For this review, take the finished solid that the model builds, in its own axes (mm). A direction names the side the tool comes from. Round coordinates to 2 decimals unless told otherwise and drop trailing zeros. Loops run counter-clockwise (first coordinate to the right, second up) from the corner with the lowest first, then second, coordinate; pieces in that order, holes last.
1) Take a section at B-B (z = -58). State the section outline as (x, y) points (3 decimals).
2) Take a section at C-C (x = 31). State the section outline as (y, z) points.
3) Insertion check: pin 1 (3 mm diameter, centred on x = -6, y = 27.5, fed in from +Z); pin 2 (8 mm diameter, centred on y = -0.5, z = -64, fed in from -X); pin 3 (3 mm diameter, centred on x = -1, z = -66, fed in from -Y). Each pin has a flat end and moves straight along its axis. Give the tip position at first contact, or say it passes through.
4) Tool access review of faces 1 (the cylindrical face through (-26, 0, 5)), 2 (the flat face through (5.25, 0, -65)), 3 (the flat face through (0, -5.25, -65)), 4 (the flat face through (-5.25, 0, -65)): name each direction out of +Z, -Z, +X, -X, +Y, -Y from which nothing blocks a thin tool from reaching the whole face with its end or side.
5) Take a section at D-D (z = 20.5). State the section outline as (x, y) points, then the cut area to 3 significant figures.
6) Mouldability with a two-part tool opening along Y and no side actions: class faces 5 (the flat face through (-24, -38, 55)), 6 (the flat face through (0, 0, -60.1)), 7 (the cylindrical face through (47.23, -1.34, 32.18)) as pulls with the +Y half, pulls with the -Y half, needs draft (parallel to the pull), parting line crosses it, or undercut.
```python
from build123d import *
from build123d.topology import SkipClean

# Parameters (mm, degrees)
SKETCH1_R           = 57
SKETCH1_R_2         = 5.175
BOSS_EXTRUDE1_DEPTH = 10
SKETCH3_R           = 2.25
BOSS_EXTRUDE2_DEPTH = 45
BOSS_EXTRUDE3_START = 60.1
SKETCH4_R           = 9.75
SKETCH4_R_2         = 5.175
BOSS_EXTRUDE3_DEPTH = 60.1
SKETCH5_W           = 10.5
SKETCH5_H           = 10.5
BOSS_EXTRUDE4_DEPTH = 10
CUT_EXTRUDE1_DEPTH  = 10
CIRPATTERN1_COUNT   = 3


with BuildPart() as part:
    # Sketch1 → Boss-Extrude1 (new body)
    with BuildSketch(Plane(origin=(0, 0, 0), x_dir=(0, 1, 0), z_dir=(0, 0, 1))):
        with Locations(Location((0, 0, 0), (0, 0, 270))):
            Circle(SKETCH1_R)
        with Locations(Location((0, 0, 0), (0, 0, 270))):
            Circle(SKETCH1_R_2, mode=Mode.SUBTRACT)
    extrude(amount=BOSS_EXTRUDE1_DEPTH)

    # Sketch3 → Boss-Extrude2 (add)
    with BuildSketch(Plane.XY.offset(10)):
        with Locations(Location((-21.418860984, 39.575654059, 0), (0, 0, 180))):
            Circle(SKETCH3_R)
    boss_extrude2 = extrude(amount=BOSS_EXTRUDE2_DEPTH)

    # Sketch4 → Boss-Extrude3 (add)
    with SkipClean():  # the faces are left unmerged after this step: merging them gives an invalid solid
        with BuildSketch(Plane(origin=(0, 0, 0), x_dir=(-1, 0, 0), z_dir=(0, 0, -1)).offset(BOSS_EXTRUDE3_START)):
            with Locations(Location((0, 0, 0), (0, 0, 180))):
                Circle(SKETCH4_R)
            Circle(SKETCH4_R_2, mode=Mode.SUBTRACT)
        extrude(amount=-BOSS_EXTRUDE3_DEPTH)

    # Sketch5 → Boss-Extrude4 (add)
    with SkipClean():  # the faces are left unmerged after this step: merging them gives an invalid solid
        with BuildSketch(Plane(origin=(0, 0, -60.1), x_dir=(-1, 0, 0), z_dir=(0, 0, -1))):
            Rectangle(SKETCH5_W, SKETCH5_H)
        extrude(amount=BOSS_EXTRUDE4_DEPTH)

    # Sketch6 → Cut-Extrude1 (cut)
    with SkipClean():  # the faces are left unmerged after this step: merging them gives an invalid solid
        with BuildSketch(Plane(origin=(0, 0, 0), x_dir=(-1, 0, 0), z_dir=(0, 0, -1))):
            with BuildLine():
                ThreePointArc((31.321270818, -21.51692344), (37.99899628, 0.276191416), (31.005191486, 21.969936298))
                ThreePointArc((31.005191486, 21.969936298), (22.640697625, 23.396555538), (21.214078385, 15.032061678))
                ThreePointArc((21.214078385, 15.032061678), (25.999313244, 0.188973074), (21.430343191, -14.722105512))
                ThreePointArc((21.430343191, -14.722105512), (22.978398041, -23.064978289), (31.321270818, -21.51692344))
            make_face()
            with BuildLine():
                ThreePointArc((-34.384548284, -16.177232126), (-18.887293866, -32.973779438), (3.441417522, -37.843845542))
                ThreePointArc((3.441417522, -37.843845542), (8.873379841, -31.325119796), (2.354654094, -25.893157476))
                ThreePointArc((2.354654094, -25.893157476), (-12.922885277, -22.561006984), (-23.526269879, -11.068632508))
                ThreePointArc((-23.526269879, -11.068632508), (-31.509708891, -8.193793114), (-34.384548284, -16.177232126))
            make_face()
            with BuildLine():
                ThreePointArc((3.531923315, 37.835506045), (-18.808372522, 33.018860112), (-34.345756916, 16.259427476))
                ThreePointArc((-34.345756916, 16.259427476), (-31.490020689, 8.269135204), (-23.499728416, 11.124871431))
                ThreePointArc((-23.499728416, 11.124871431), (-12.868886462, 22.591851656), (2.41657911, 25.887451505))
                ThreePointArc((2.41657911, 25.887451505), (8.948278483, 31.303806673), (3.531923315, 37.835506045))
            make_face()
        extrude(amount=-CUT_EXTRUDE1_DEPTH, mode=Mode.SUBTRACT)

    # CirPattern1: Boss-Extrude2 ×3 about axis
    with SkipClean():  # the faces are left unmerged after this step: merging them gives an invalid solid
        cirpattern1_axis = Axis((0, 0, 0), (0, 0, 1))
        for i in range(1, CIRPATTERN1_COUNT):
            add(boss_extrude2.rotate(cirpattern1_axis, i * 360 / CIRPATTERN1_COUNT))


solid = part.part
```
Response:
1. outline: circle Ø19.5 at (0, 0); hole circle Ø10.35 at (0, 0)
2. outline: (-47.83, 0) - (-21.98, 0) - (-21.98, 10) - (-47.83, 10) - close; (-7.98, 0) - (8.06, 0) - (8.06, 10) - (-7.98, 10) - close; (21.98, 0) - (47.83, 0) - (47.83, 10) - (21.98, 10) - close
3. pin 1: stops at z = 10
3. pin 2: stops at x = -9.75
3. pin 3: stops at y = -5.25
4. face 1: +Z, -Z
4. face 2: -Z, +X, +Y, -Y
4. face 3: -Z, +X, -X, -Y
4. face 4: -Z, -X, +Y, -Y
5. outline: circle Ø4.5 at (-23.56, -38.34); circle Ø4.5 at (-21.42, 39.58); circle Ø4.5 at (44.98, -1.24)
5. area: 47.7 mm2
6. face 5: needs draft
6. face 6: undercut
6. face 7: parting line crosses it
